from build123d import *

# Parameters (mm, degrees)
SKETCH_1_R      = 14
SKETCH_1_R_2    = 1.5
EXTRUDE_1_DEPTH = 4
SKETCH_2_R      = 7.5
SKETCH_2_R_2    = 2.5
EXTRUDE_2_DEPTH = 7


with BuildPart() as part:
    # 草图1 → 凸台-拉伸1 (new body)
    with BuildSketch(Plane(origin=(0, 0, 0), x_dir=(1, 0, 0), z_dir=(0, 1, 0))):
        with Locations(Location((0, 0, 0), (0, 0, 270))):
            Circle(SKETCH_1_R)
        with Locations(Location((0, 11.5, 0), (0, 0, 270))):
            Circle(SKETCH_1_R_2, mode=Mode.SUBTRACT)
        with Locations(Location((9.959292144, -5.75, 0), (0, 0, 270))):
            Circle(SKETCH_1_R_2, mode=Mode.SUBTRACT)
        with Locations(Location((-9.959292144, -5.75, 0), (0, 0, 270))):
            Circle(SKETCH_1_R_2, mode=Mode.SUBTRACT)
    extrude(amount=EXTRUDE_1_DEPTH)

    # 草图2 → 凸台-拉伸2 (add)
    with BuildSketch(Plane(origin=(0, 4, 0), x_dir=(1, 0, 0), z_dir=(0, 1, 0))):
        with Locations(Location((0, 0, 0), (0, 0, 270))):
            Circle(SKETCH_2_R)
        with Locations(Location((0, 0, 0), (0, 0, 270))):
            Circle(SKETCH_2_R_2, mode=Mode.SUBTRACT)
    extrude(amount=EXTRUDE_2_DEPTH)


solid = part.part
Design review of the part built by this model. Coordinates are the model's own, in mm. A direction names the side the tool comes from. Round coordinates to 2 decimals unless told otherwise and drop trailing zeros. Loops run counter-clockwise (first coordinate to the right, second up) from the corner with the lowest first, then second, coordinate; pieces in that order, holes last. Notation, with made-up numbers: M -27,0.5 L 2,0.5 A22 cw 2,15.5 Z; hole C -4.75,42.25 d4. An arc over 180 degrees is marked long. Answer as a JSON object with one key per item and string values.
Item 1: We need section C-C on y = 5.75. Give the boundary of the cut face in (x, z).
Answer sheet:
{"outline": "C 0,0 d15; hole C 0,0 d5"}
Item 2: Machinability: for faces 4 (the flat face through (2, 11, -2)), 5 (the cylindrical face through (0.33, 7.451, -7.493)), which of the approach directions +Z, -Z, +X, -X, +Y, -Y give a long, thin tool a straight path to every point of the face, cutting with its end or side? Answer none if there is none.
Answer sheet:
{"face 4": "+Z, -Z, +X, -X, +Y", "face 5": "+Y"}
Item 3: We need section A-A on x = 0. Give the boundary of the cut face in (y, z), and give its area (3 significant figures).
Answer sheet:
{"outline": "M 0,-14 L 4,-14 L 4,-13 L 0,-13 Z; M 0,-10 L 4,-10 L 4,-7.5 L 11,-7.5 L 11,-2.5 L 4,-2.5 L 4,2.5 L 11,2.5 L 11,7.5 L 4,7.5 L 4,14 L 0,14 Z", "area": "170 mm^2"}
Item 4: The part is to be moulded in two halves that separate along X. For faces 1 (the cylindrical face through (-13.67, 1.97, -3.03)), 2 (the cylindrical face through (0, 2, -13)), 3 (the flat face through (-6, 4, 6)), say which applies: pulls with the +X half, pulls with the -X half, needs draft (parallel to the pull), parting line crosses it, or undercut.
Answer sheet:
{"face 1": "parting line crosses it", "face 2": "undercut", "face 3": "needs draft"}
Item 5: Clearance check with flat-ended pins moving along their axes: P1, Ø3.5, axis at x = -9.96, z = 5.75, coming from the +Y side; P2, Ø4, axis at x = 10.5, y = 8.5, coming from the -Z side; P3, Ø5, axis at x = -10.5, y = 5.5, coming from the +Z side; P4, Ø1.5, axis at x = -4.5, y = 4.5, coming from the -Z side. State where each tip first meets the part, or that it passes through.
Answer sheet:
{"P1": "stops at y = 4", "P2": "passes through", "P3": "stops at z = 11.12", "P4": "stops at z = -13.43"}
Item 6: We need section B-B on z = -11.5. Give the boundary of the cut face in (x, y).
Answer sheet:
{"outline": "M -7.98,0 L -1.5,0 L -1.5,4 L -7.98,4 Z; M 1.5,0 L 7.98,0 L 7.98,4 L 1.5,4 Z"}
Item 7: We need section D-D on z = 5.75. Give the boundary of the cut face in (x, y).
Answer sheet:
{"outline": "M -12.76,0 L -11.46,0 L -11.46,4 L -12.76,4 Z; M -8.46,0 L 8.46,0 L 8.46,4 L 4.82,4 L 4.82,11 L -4.82,11 L -4.82,4 L -8.46,4 Z; M 11.46,0 L 12.76,0 L 12.76,4 L 11.46,4 Z"}
Item 8: Wall thickness on L1, parallel to Y at x = -10.75, z = -6.75; L2, parallel to X at y = 2.25, z = 5; L3, parallel to Z at x = 2.25, y = 6.5: over which ranges is each line inside the solid? List them lowest first. Write a range as from..to.
Answer sheet:
{"L1": "y = 0..4", "L2": "x = -13.08..-11.26, -8.66..8.66, 11.26..13.08", "L3": "z = -7.15..-1.09, 1.09..7.15"}
